from build123d import *

# Parameters (mm, degrees)
SKETCH1_R                  = 4
SKETCH1_R_2                = 1.5
BASE_FLANGE1_DEPTH         = 2
SKETCHED_START             = -92.5
SKETCHED_BEND1_OUTLINE_W   = 2
SKETCHED_BEND1_OUTLINE_H   = 25
SKETCHED_BEND1_DEPTH       = 65
SKETCHED_START_2           = 27.5
SKETCHED_BEND1_2_OUTLINE_W = 2
SKETCHED_BEND1_2_OUTLINE_H = 25
SKETCHED_BEND1_2_DEPTH     = 65
SKETCHED_START_3           = -27.5
SKETCHED_BEND1_3_OUTLINE_R = 1.5
SKETCHED_BEND1_3_DEPTH     = 2.7366
SKETCHED_START_4           = 24.7634
SKETCHED_BEND1_4_OUTLINE_R = 1.5
SKETCHED_BEND1_4_DEPTH     = 2.7366
SKETCHED_BEND1_5_DEPTH     = 2
SKETCHED_START_5           = 25.5
SKETCHED_BEND1_6_DEPTH     = 2
SKETCHED_START_6           = -12.5
SKETCHED_BEND1_7_DEPTH     = 25


with BuildPart() as part:
    # Base-Flange1: sheet metal written as solids
    # Sketch1 → Base-Flange1 (new body)
    with BuildSketch(Plane(origin=(0, 0, 0), x_dir=(1, 0, 0), z_dir=(0, 1, 0))):
        with BuildLine():
            Line((-92.5, -0.001), (-92.5, 0.001))
            ThreePointArc((-92.5, 0.001), (-88.839127658, 8.839127658), (-80.001, 12.5))
            Line((-80.001, 12.5), (80.001, 12.5))
            ThreePointArc((80.001, 12.5), (88.839127658, 8.839127658), (92.5, 0.001))
            Line((92.5, 0.001), (92.5, -0.001))
            ThreePointArc((92.5, -0.001), (88.839127658, -8.839127658), (80.001, -12.5))
            Line((80.001, -12.5), (-80.001, -12.5))
            ThreePointArc((-80.001, -12.5), (-88.839127658, -8.839127658), (-92.5, -0.001))
        make_face()
        with Locations(Location((0, 0, 0), (0, 0, 270))):
            Circle(SKETCH1_R, mode=Mode.SUBTRACT)
        with Locations(Location((0, 7.5, 0), (0, 0, 270))):
            Circle(SKETCH1_R_2, mode=Mode.SUBTRACT)
        with Locations(Location((7.5, 0, 0), (0, 0, 270))):
            Circle(SKETCH1_R_2, mode=Mode.SUBTRACT)
        with Locations(Location((0, -7.5, 0), (0, 0, 270))):
            Circle(SKETCH1_R_2, mode=Mode.SUBTRACT)
        with Locations(Location((-7.5, 0, 0), (0, 0, 270))):
            Circle(SKETCH1_R_2, mode=Mode.SUBTRACT)
        with Locations(Location((72.501, 0.001, 0), (0, 0, 270))):
            Circle(SKETCH1_R_2, mode=Mode.SUBTRACT)
        with Locations(Location((80.001, 0.001, 0), (0, 0, 270))):
            Circle(SKETCH1_R, mode=Mode.SUBTRACT)
        with Locations(Location((80.001, -7.499, 0), (0, 0, 270))):
            Circle(SKETCH1_R_2, mode=Mode.SUBTRACT)
        with Locations(Location((87.501, 0.001, 0), (0, 0, 270))):
            Circle(SKETCH1_R_2, mode=Mode.SUBTRACT)
        with Locations(Location((80.001, 7.501, 0), (0, 0, 270))):
            Circle(SKETCH1_R_2, mode=Mode.SUBTRACT)
        with Locations(Location((-80.001, 7.499, 0), (0, 0, 270))):
            Circle(SKETCH1_R_2, mode=Mode.SUBTRACT)
        with Locations(Location((-87.501, -0.001, 0), (0, 0, 270))):
            Circle(SKETCH1_R_2, mode=Mode.SUBTRACT)
        with Locations(Location((-80.001, -0.001, 0), (0, 0, 270))):
            Circle(SKETCH1_R, mode=Mode.SUBTRACT)
        with Locations(Location((-72.501, -0.001, 0), (0, 0, 270))):
            Circle(SKETCH1_R_2, mode=Mode.SUBTRACT)
        with Locations(Location((-80.001, -7.501, 0), (0, 0, 270))):
            Circle(SKETCH1_R_2, mode=Mode.SUBTRACT)
        with Locations(Location((-62.501, -0.001, 0), (0, 0, 270))):
            Circle(SKETCH1_R_2, mode=Mode.SUBTRACT)
        with Locations(Location((-45.501, -0.001, 0), (0, 0, 270))):
            Circle(SKETCH1_R_2, mode=Mode.SUBTRACT)
        with Locations(Location((45.501, -0.001, 0), (0, 0, 90))):
            Circle(SKETCH1_R_2, mode=Mode.SUBTRACT)
        with Locations(Location((62.501, -0.001, 0), (0, 0, 90))):
            Circle(SKETCH1_R_2, mode=Mode.SUBTRACT)
        with Locations(Location((19.5, 0, 0), (0, 0, 270))):
            Circle(SKETCH1_R_2, mode=Mode.SUBTRACT)
        with Locations(Location((-19.5, 0, 0), (0, 0, 90))):
            Circle(SKETCH1_R_2, mode=Mode.SUBTRACT)
    extrude(amount=-BASE_FLANGE1_DEPTH)

    # Sketched Bend1: read off the stored shape, not the designer's step
    # Sketched Bend1 outline → Sketched Bend1 (cut)
    with BuildSketch(Plane.YZ.offset(SKETCHED_START)):
        with Locations((-1, 0)):
            Rectangle(SKETCHED_BEND1_OUTLINE_W, SKETCHED_BEND1_OUTLINE_H)
    extrude(amount=SKETCHED_BEND1_DEPTH, mode=Mode.SUBTRACT)

    # Sketched Bend1 2 outline → Sketched Bend1 2 (cut)
    with BuildSketch(Plane.YZ.offset(SKETCHED_START_2)):
        with Locations((-1, 0)):
            Rectangle(SKETCHED_BEND1_2_OUTLINE_W, SKETCHED_BEND1_2_OUTLINE_H)
    extrude(amount=SKETCHED_BEND1_2_DEPTH, mode=Mode.SUBTRACT)

    # Sketched Bend1 3 outline → Sketched Bend1 3 (add)
    with BuildSketch(Plane.YZ.offset(SKETCHED_START_3)):
        with BuildLine():
            Line((0, 12.5), (0, -12.5))
            Line((0, -12.5), (53.246355099, -12.5))
            ThreePointArc((53.246355099, -12.5), (62.084482757, -8.839127658), (65.745355099, -0.001))
            Line((65.745355099, -0.001), (65.745355099, 0.001))
            ThreePointArc((65.745355099, 0.001), (62.084482757, 8.839127658), (53.246355099, 12.5))
            Line((53.246355099, 12.5), (0, 12.5))
        make_face()
        with BuildLine():
            ThreePointArc((54.746353766, -7.499000002), (53.246855098, -9.000999917), (51.746355432, -7.5))
            ThreePointArc((51.746355432, -7.5), (53.245855099, -5.999000083), (54.746353766, -7.499000002))
        make_face(mode=Mode.SUBTRACT)
        with Locations((18.746355099, 0.001)):
            Circle(SKETCHED_BEND1_3_OUTLINE_R, mode=Mode.SUBTRACT)
        with Locations((35.746355099, 0.001)):
            Circle(SKETCHED_BEND1_3_OUTLINE_R, mode=Mode.SUBTRACT)
        with BuildLine():
            ThreePointArc((47.246353766, 0.000999998), (45.746855098, -1.500999917), (44.246355432, 0))
            ThreePointArc((44.246355432, 0), (45.745855099, 1.500999917), (47.246353766, 0.000999998))
        make_face(mode=Mode.SUBTRACT)
        with BuildLine():
            ThreePointArc((57.246354599, 0.001), (53.246855099, -4.000999969), (49.246355224, 0))
            ThreePointArc((49.246355224, 0), (53.245855099, 4.000999969), (57.246354599, 0.001))
        make_face(mode=Mode.SUBTRACT)
        with BuildLine():
            ThreePointArc((62.246353766, 0.000999998), (60.746855098, -1.500999917), (59.246355432, 0))
            ThreePointArc((59.246355432, 0), (60.745855099, 1.500999917), (62.246353766, 0.000999998))
        make_face(mode=Mode.SUBTRACT)
        with BuildLine():
            ThreePointArc((54.746353766, 7.500999998), (53.246855098, 5.999000083), (51.746355432, 7.5))
            ThreePointArc((51.746355432, 7.5), (53.245855099, 9.000999917), (54.746353766, 7.500999998))
        make_face(mode=Mode.SUBTRACT)
    extrude(amount=SKETCHED_BEND1_3_DEPTH)

    # Sketched Bend1 4 outline → Sketched Bend1 4 (add)
    with BuildSketch(Plane.YZ.offset(SKETCHED_START_4)):
        with BuildLine():
            Line((0, 12.5), (0, -12.5))
            Line((0, -12.5), (53.246355099, -12.5))
            ThreePointArc((53.246355099, -12.5), (62.084482757, -8.839127658), (65.745355099, -0.001))
            Line((65.745355099, -0.001), (65.745355099, 0.001))
            ThreePointArc((65.745355099, 0.001), (62.084482757, 8.839127658), (53.246355099, 12.5))
            Line((53.246355099, 12.5), (0, 12.5))
        make_face()
        with BuildLine():
            ThreePointArc((54.746353766, -7.499000002), (53.246855098, -9.000999917), (51.746355432, -7.5))
            ThreePointArc((51.746355432, -7.5), (53.245855099, -5.999000083), (54.746353766, -7.499000002))
        make_face(mode=Mode.SUBTRACT)
        with Locations((18.746355099, 0.001)):
            Circle(SKETCHED_BEND1_4_OUTLINE_R, mode=Mode.SUBTRACT)
        with Locations((35.746355099, 0.001)):
            Circle(SKETCHED_BEND1_4_OUTLINE_R, mode=Mode.SUBTRACT)
        with BuildLine():
            ThreePointArc((47.246353766, 0.000999998), (45.746855098, -1.500999917), (44.246355432, 0))
            ThreePointArc((44.246355432, 0), (45.745855099, 1.500999917), (47.246353766, 0.000999998))
        make_face(mode=Mode.SUBTRACT)
        with BuildLine():
            ThreePointArc((57.246354599, 0.001), (53.246855099, -4.000999969), (49.246355224, 0))
            ThreePointArc((49.246355224, 0), (53.245855099, 4.000999969), (57.246354599, 0.001))
        make_face(mode=Mode.SUBTRACT)
        with BuildLine():
            ThreePointArc((62.246353766, 0.000999998), (60.746855098, -1.500999917), (59.246355432, 0))
            ThreePointArc((59.246355432, 0), (60.745855099, 1.500999917), (62.246353766, 0.000999998))
        make_face(mode=Mode.SUBTRACT)
        with BuildLine():
            ThreePointArc((54.746353766, 7.500999998), (53.246855098, 5.999000083), (51.746355432, 7.5))
            ThreePointArc((51.746355432, 7.5), (53.245855099, 9.000999917), (54.746353766, 7.500999998))
        make_face(mode=Mode.SUBTRACT)
    extrude(amount=SKETCHED_BEND1_4_DEPTH)

    # Sketched Bend1 5 outline → Sketched Bend1 5 (add)
    with BuildSketch(Plane.YZ.offset(SKETCHED_START_3)):
        with BuildLine():
            ThreePointArc((44.246355432, 0), (45.745855099, -1.500999917), (47.246355099, -0.001))
            ThreePointArc((47.246355099, -0.001), (45.7458551, -1.498999917), (44.246355432, 0))
        make_face()
        with BuildLine():
            ThreePointArc((51.746355432, 7.5), (53.245855099, 5.999000083), (54.746355099, 7.499))
            ThreePointArc((54.746355099, 7.499), (53.2458551, 6.001000083), (51.746355432, 7.5))
        make_face()
        with BuildLine():
            ThreePointArc((59.246355432, 0), (60.745855099, -1.500999917), (62.246355099, -0.001))
            ThreePointArc((62.246355099, -0.001), (60.7458551, -1.498999917), (59.246355432, 0))
        make_face()
        with BuildLine():
            ThreePointArc((51.746355432, -7.5), (53.245855099, -9.000999917), (54.746355099, -7.501))
            ThreePointArc((54.746355099, -7.501), (53.2458551, -8.998999917), (51.746355432, -7.5))
        make_face()
        with BuildLine():
            ThreePointArc((49.246355224, 0), (53.245855099, -4.000999969), (57.246355099, -0.001))
            ThreePointArc((57.246355099, -0.001), (53.245855099, -3.998999969), (49.246355224, 0))
        make_face()
    extrude(amount=SKETCHED_BEND1_5_DEPTH)

    # Sketched Bend1 6 outline → Sketched Bend1 6 (add)
    with BuildSketch(Plane.YZ.offset(SKETCHED_START_5)):
        with BuildLine():
            ThreePointArc((44.246355432, 0), (45.7458551, 1.498999917), (47.246353766, 0.000999998))
            ThreePointArc((47.246353766, 0.000999998), (45.745855099, 1.500999917), (44.246355432, 0))
        make_face()
        with BuildLine():
            ThreePointArc((51.746355432, 7.5), (53.2458551, 8.998999917), (54.746353766, 7.500999998))
            ThreePointArc((54.746353766, 7.500999998), (53.245855099, 9.000999917), (51.746355432, 7.5))
        make_face()
        with BuildLine():
            ThreePointArc((59.246355432, 0), (60.7458551, 1.498999917), (62.246353766, 0.000999998))
            ThreePointArc((62.246353766, 0.000999998), (60.745855099, 1.500999917), (59.246355432, 0))
        make_face()
        with BuildLine():
            ThreePointArc((51.746355432, -7.5), (53.2458551, -6.001000083), (54.746353766, -7.499000002))
            ThreePointArc((54.746353766, -7.499000002), (53.245855099, -5.999000083), (51.746355432, -7.5))
        make_face()
        with BuildLine():
            ThreePointArc((49.246355224, 0), (53.245855099, 3.998999969), (57.246354599, 0.001))
            ThreePointArc((57.246354599, 0.001), (53.245855099, 4.000999969), (49.246355224, 0))
        make_face()
    extrude(amount=SKETCHED_BEND1_6_DEPTH)

    # Sketched Bend1 7 outline → Sketched Bend1 7 (cut)
    with BuildSketch(Plane.XY.offset(SKETCHED_START_6)):
        with BuildLine():
            Line((25.5, 0.7366), (25.5, 65.745355099))
            Line((25.5, 65.745355099), (24.7634, 65.745355099))
            Line((24.7634, 65.745355099), (24.7634, 0))
            ThreePointArc((24.7634, 0), (25.284254855, 0.215745145), (25.5, 0.7366))
        make_face()
        with BuildLine():
            Line((-24.7634, 65.745355099), (-25.5, 65.745355099))
            Line((-25.5, 65.745355099), (-25.5, 0.7366))
            ThreePointArc((-25.5, 0.7366), (-25.284254855, 0.215745145), (-24.7634, 0))
            Line((-24.7634, 0), (-24.7634, 65.745355099))
        make_face()
        with BuildLine():
            Line((-27.5, -2), (-24.7634, -2))
            ThreePointArc((-24.7634, -2), (-26.698468417, -1.198468417), (-27.5, 0.7366))
            Line((-27.5, 0.7366), (-27.5, -2))
        make_face()
        with BuildLine():
            ThreePointArc((27.5, 0.7366), (26.698468417, -1.198468417), (24.7634, -2))
            Line((24.7634, -2), (27.5, -2))
            Line((27.5, -2), (27.5, 0.7366))
        make_face()
    extrude(amount=SKETCHED_BEND1_7_DEPTH, mode=Mode.SUBTRACT)


solid = part.part
Source: CAD feature listing. Evaluate the final solid. Frame: model axes, mm. A direction names the side the tool comes from. Coordinates: 2 decimals unless noted, no trailing zeros. Order: outer loops, then holes, each group sorted by start corner. A loop starts at its lowest first (then second) coordinate and runs counter-clockwise, first axis right, second up. Notation, with made-up numbers: M -1.75,28.25 L 52.25,28.25 A10 cw 52.25,43.25 Z; hole C -30,27 d1. An arc over 180 degrees is marked long. Write each question's results on one line, items separated by ' | '. Start each with the question number.
1. Material intervals for L1, parallel to X at y = 53.5, z = -11; L2, parallel to X at y = -1.35, z = 0; L3, parallel to X at y = -1.25, z = 0, sorted ascending.
2. Section B-B, the plane x = 19.5. Return the cut outline in (y, z), then the cut area to 3 significant figures.
3. Section C-C, the plane y = 55.5. Return the cut outline in (x, z), then the cut area to 3 significant figures.
4. Reachability of faces 1 (the face through (-26.514, 61.987, -8.936)), 2 (the face through (-25.5, 34, 0)) from +Z, -Z, +X, -X, +Y, -Y: full face, straight path, thin tool, end or side. Return the list, or none.
5. Section D-D, the plane z = 10.5. Return the cut outline in (x, y).
6. Pin query (flat end, axial travel): pin 1 (4 mm diameter, centred on x = -7.5, z = 0, fed in from +Y); pin 2 (1.8 mm diameter, centred on y = 18.75, z = 0, fed in from -X). Return the tip coordinate at first contact, or that it passes through.
7. Section A-A, the plane y = 30. Return the cut outline in (x, z), then the cut area to 3 significant figures.
8. Draft query along X for faces 3 (the face through (-5, 0, 0)), 4 (the face through (0, -1, 6)), 5 (the face through (26.486, 59.316, 0.451)), 6 (the face through (26.72, -1.177, -0.175)). Return one class per face: +X half, -X half, draft (parallel to the pull), parting line (faces both ways), or undercut.
Solution:
1) L1: -27.5 to -25.5, 25.5 to 27.5 | L2: -26.53 to -21, -18 to -9, -6 to -4, 4 to 6, 9 to 18, 21 to 26.53 | L3: -26.65 to -21, -18 to -9, -6 to -4, 4 to 6, 9 to 18, 21 to 26.65
2) outline: M -2,-12.5 L 0,-12.5 L 0,-1.5 L -2,-1.5 Z; M -2,1.5 L 0,1.5 L 0,12.5 L -2,12.5 Z | area: 44.0 mm²
3) outline: M -27.5,-12.3 L -25.5,-12.3 L -25.5,-3.3 L -27.5,-3.3 Z; M -27.5,3.31 L -25.5,3.31 L -25.5,12.3 L -27.5,12.3 Z; M 25.5,-12.3 L 27.5,-12.3 L 27.5,-3.31 L 25.5,-3.31 Z; M 25.5,3.3 L 27.5,3.3 L 27.5,12.3 L 25.5,12.3 Z | area: 71.9 mm²
4) face 1: -Z, +X, -X, +Y | face 2: +Z, -Z, +Y
5) outline: M -27.5,0.74 A2.74 ccw -24.76,-2 L 24.76,-2 A2.74 ccw 27.5,0.74 L 27.5,60.03 L 25.5,60.03 L 25.5,0.74 A0.74 cw 24.76,0 L -24.76,0 A0.74 cw -25.5,0.74 L -25.5,60.03 L -27.5,60.03 Z
6) pin 1: y = 0 | pin 2: through
7) outline: M -27.5,-12.5 L -25.5,-12.5 L -25.5,12.5 L -27.5,12.5 Z; M 25.5,-12.5 L 27.5,-12.5 L 27.5,12.5 L 25.5,12.5 Z | area: 100 mm²
8) face 3: undercut | face 4: undercut | face 5: draft | face 6: +X half
